```python
from build123d import *

# Parameters (mm, degrees)
AUFSATZ_LINEAR_AUSTRAGEN1_DEPTH  = 25
SCHNITT_LINEAR_AUSTRAGEN1_DEPTH  = 12
F_25_0_25_DURCHMESSER_BOHRUNG1_D = 25
M6_GEWINDEBOHRUNG1_D             = 5
M6_GEWINDEBOHRUNG1_DEPTH         = 17
M6_GEWINDEBOHRUNG1_TIP           = 1.502151548
M12_GEWINDEBOHRUNG1_D            = 10.2
M12_GEWINDEBOHRUNG1_DEPTH        = 25
M12_GEWINDEBOHRUNG1_TIP          = 3.064389157


with BuildPart() as part:
    # Skizze1 → Aufsatz-Linear austragen1 (new, symmetric)
    with BuildSketch(Plane.XY):
        with BuildLine():
            Line((0, 0), (120.12882084, 61.208691436))
            Line((120.12882084, 61.208691436), (140.303776199, 54.653451069))
            Line((140.303776199, 54.653451069), (149.383586194, 36.833320585))
            Line((149.383586194, 36.833320585), (142.828345827, 16.658365227))
            Line((142.828345827, 16.658365227), (121.444189247, 5.762593233))
            ThreePointArc((121.444189247, 5.762593233), (103.556160862, 5.62679743), (92.931980473, -8.765102759))
            Line((92.931980473, -8.765102759), (0, -56.116311882))
            Line((0, -56.116311882), (0, 0))
        make_face()
    extrude(amount=AUFSATZ_LINEAR_AUSTRAGEN1_DEPTH, both=True)

    # Skizze2 → Schnitt-Linear austragen1 (cut, symmetric)
    with BuildSketch(Plane.XY):
        Polygon((133.493918703, 68.018548932), (81.8155403, 41.687099947), (104.515065287, -2.863226262), (156.19344369, 23.468222723), align=None)
    extrude(amount=SCHNITT_LINEAR_AUSTRAGEN1_DEPTH, both=True, mode=Mode.SUBTRACT)

    # Ø25.0 (25) Durchmesser Bohrung1 (through all)
    with Locations(Plane.XY.offset(25)):
        with Locations((127.023550713, 36.663575833)):
            Hole(F_25_0_25_DURCHMESSER_BOHRUNG1_D / 2)

    # M6 Gewindebohrung1
    with Locations(Plane(origin=(133.493918703, 68.018548932, 0), x_dir=(0, 0, -1), z_dir=(0.8910065241883688, 0.4539904997395451, 0))):
        with Locations((-18.5, -25)):
            Hole(M6_GEWINDEBOHRUNG1_D / 2, depth=M6_GEWINDEBOHRUNG1_DEPTH)
            with Locations((0, 0, -(M6_GEWINDEBOHRUNG1_DEPTH + M6_GEWINDEBOHRUNG1_TIP / 2))):  # 118° drill point
                Cone(0, M6_GEWINDEBOHRUNG1_D / 2, M6_GEWINDEBOHRUNG1_TIP, mode=Mode.SUBTRACT)

    # M12 Gewindebohrung1
    with Locations(Plane.ZY):
        with Locations((-12.5, -12), (12.5, -12), (0, -32)):
            Hole(M12_GEWINDEBOHRUNG1_D / 2, depth=M12_GEWINDEBOHRUNG1_DEPTH)
            with Locations((0, 0, -(M12_GEWINDEBOHRUNG1_DEPTH + M12_GEWINDEBOHRUNG1_TIP / 2))):  # 118° drill point
                Cone(0, M12_GEWINDEBOHRUNG1_D / 2, M12_GEWINDEBOHRUNG1_TIP, mode=Mode.SUBTRACT)


solid = part.part
```
The model under review builds one solid part; all positions refer to its coordinate system, in mm. A direction names the side the tool comes from. Coordinates: 2 decimals unless noted, no trailing zeros. Order: outer loops, then holes, each group sorted by start corner. A loop starts at its lowest first (then second) coordinate and runs counter-clockwise, first axis right, second up. Notation, with made-up numbers: (45, 23.25) -> (76, 23.25) arc R27 ccw to (76, 60.25) -> close; hole circle Ø6 at (-24, 74.25). An arc over 180 degrees is marked (long way). Answer in a Markdown table with one row per item. Add a question column.
Item 1: We need section C-C on y = -43. Write out the cut boundary in (x, z), plus the area to 3 significant figures.
Item 2: Clearance check with flat-ended pins moving along their axes: pin 1 (16.5 mm diameter, centred on y = -12, z = -12.5, fed in from +X); pin 2 (6 mm diameter, centred on y = 36, z = -5, fed in from +X); pin 3 (8 mm diameter, centred on y = -40.5, z = 14.5, fed in from -X); pin 4 (10 mm diameter, centred on y = -2.5, z = 11, fed in from +X). State where each tip first meets the part, or that it passes through.
Item 3: Mouldability with a two-part tool opening along Y and no side actions: class faces 4 (the flat face through (91.267, 23.139, 0.168)), 5 (the cylindrical face through (12.675, -10.468, -17.364)), 6 (the flat face through (115, 27, 12)) as +Y half, -Y half, draft (parallel to the pull), parting line (faces both ways), or undercut.
Item 4: We need section A-A on z = -21. Write out the cut boundary in (x, y).
Item 5: We need section D-D on x = 42. Write out the cut boundary in (y, z).
Item 6: To check wall thickness, follow probe 1 along Z at (x, y) = (6.5, -12); probe 2 along Z at (x, y) = (120.5, 14.5); probe 3 along Y at (x, z) = (20, 1.5). State the ranges of each line that lie inside material, in increasing order.
Item 7: We need section B-B on x = 91. Write out the cut boundary in (y, z).
Item 8: Machinability: for faces 1 (the flat face through (115, 27, -12)), 2 (the flat face through (47.117, -32.109, 0.35)), 3 (the cylindrical face through (12.675, -10.468, 7.636)), which of the approach directions +Z, -Z, +X, -X, +Y, -Y give a long, thin tool a straight path to every point of the face, cutting with its end or side? Answer none if there is none.
Final values:
| question | item | result |
|---|---|---|
| 1 | outline | (0, -25) -> (25.74, -25) -> (25.74, 25) -> (0, 25) -> close |
| 1 | area | 1,290 mm2 |
| 2 | pin 1 | stops at x = 94.51 |
| 2 | pin 2 | stops at x = 86.24 |
| 2 | pin 3 | stops at x = 0 |
| 2 | pin 4 | stops at x = 99.07 |
| 3 | face 4 | +Y half |
| 3 | face 5 | undercut |
| 3 | face 6 | draft |
| 4 | outline | (0, -56.12) -> (92.93, -8.77) arc R20 cw to (121.44, 5.76) -> (142.83, 16.66) -> (149.38, 36.83) -> (140.3, 54.65) -> (120.13, 61.21) -> (0, 0) -> close; hole circle Ø25 at (127.02, 36.66) |
| 5 | outline | (-34.72, -25) -> (21.4, -25) -> (21.4, 25) -> (-34.72, 25) -> close |
| 6 | probe 1 | z = -25 to -17.6, -7.4 to 7.4, 17.6 to 25 |
| 6 | probe 2 | z = -25 to -12, 12 to 25 |
| 6 | probe 3 | y = -45.93 to -36.87, -27.13 to 10.19 |
| 7 | outline | (-9.75, -25) -> (46.37, -25) -> (46.37, -12) -> (23.66, -12) -> (23.66, 12) -> (46.37, 12) -> (46.37, 25) -> (-9.75, 25) -> close |
| 8 | face 1 | +X, +Y |
| 8 | face 2 | +Z, -Z, +X, -Y |
| 8 | face 3 | -X |
